from build123d import *

# Parameters (mm, degrees)
F0_R          = 19.05
F1_DEPTH      = 63.5
F3_DEPTH      = 15.875
F3_DEPTH_BACK = 4.7752
F4_R          = 6.096
F5_DEPTH      = 61.9262
F8_DEPTH      = 2.38125


with BuildPart() as f1:
    # F0 (on Front) → F1 (new body)
    with BuildSketch(Plane.XZ):
        with BuildLine():
            Line((69.85, 28.575), (0, 28.575))
            ThreePointArc((0, 28.575), (-19.345366451, -21.0306305629), (28.4756083945, 2.38125))
            ThreePointArc((28.4756083945, 2.38125), (30.9572676717, 9.6234554837), (37.9674778593, 12.7))
            Line((37.9674778593, 12.7), (69.85, 12.7))
            Line((69.85, 12.7), (69.85, 28.575))
        make_face()
        Circle(F0_R, mode=Mode.SUBTRACT)
    extrude(amount=F1_DEPTH)

    # F2 (on face) → F3 (join, two sides)
    with BuildSketch(Plane.XY.offset(28.575)) as f3_sk:
        with BuildLine():
            ThreePointArc((76.1491554441, -1.6722785358), (73.1086759125, -0.4251871176), (69.85, 0))
            ThreePointArc((69.85, 0), (60.8697438789, -3.7197438789), (57.15, -12.7))
            Line((57.15, -12.7), (57.15, -31.75))
            Line((57.15, -31.75), (57.15, -50.8))
            ThreePointArc((57.15, -50.8), (60.8697438789, -59.7802561211), (69.85, -63.5))
            ThreePointArc((69.85, -63.5), (73.1086759125, -63.0748128824), (76.1491554441, -61.8277214642))
            Line((76.1491554441, -61.8277214642), (109.4993554441, -42.7777214642))
            ThreePointArc((109.4993554441, -42.7777214642), (114.1840352623, -38.1253715915), (115.9002, -31.75))
            ThreePointArc((115.9002, -31.75), (114.1840352623, -25.3746284085), (109.4993554441, -20.7222785358))
            Line((109.4993554441, -20.7222785358), (76.1491554441, -1.6722785358))
        make_face()
    extrude(amount=-F3_DEPTH)
    extrude(f3_sk.sketch, amount=F3_DEPTH_BACK)

    # F4 (on face) → F5 (cut, through all)
    with BuildSketch(Plane.XY.offset(33.3502)):
        with Locations((69.85, -12.7)):
            Circle(F4_R)
        with Locations((69.85, -50.8)):
            Circle(F4_R)
        with Locations((103.2002, -31.75)):
            Circle(F4_R)
    extrude(amount=-F5_DEPTH, mode=Mode.SUBTRACT)

    # F7 (on offset) → F8 (join, symmetric)
    with BuildSketch(Plane.XZ.offset(31.75)):
        with BuildLine():
            ThreePointArc((28.4756083945, 2.38125), (25.7719232537, -12.3425522809), (15.9950252975, -23.6788891364))
            Line((15.9950252975, -23.6788891364), (69.85, 12.7))
            Line((69.85, 12.7), (37.9674778593, 12.7))
            ThreePointArc((37.9674778593, 12.7), (30.9572676717, 9.6234554837), (28.4756083945, 2.38125))
        make_face()
    extrude(amount=F8_DEPTH, both=True)


solid = f1.part
Input: part model. Units: mm. Frame: model coordinates. A direction names the side the tool comes from. Coordinates: 2 decimals unless noted, no trailing zeros. Loops run counter-clockwise (first coordinate to the right, second up) from the corner with the lowest first, then second, coordinate; pieces in that order, holes last.
(1) Section B-B on y = -59. Return the cut outline in (x, z) (3 decimals).
(2) Section D-D on y = -35.5. Return the cut outline in (x, z) (3 decimals), then the cut area to 3 significant figures.
(3) Pull-direction query (Y, two-part tool) for faces 1 (the face through (75.481, -53.135, 23.17)), 2 (the face through (92.591, -52.436, 22.881)), 3 (the face through (80, -31, 33.35)); classes: released by +Y, released by -Y, zero draft, split by the parting line, or undercut.
(4) Material intervals for probe 1 along Y at (x, z) = (69.85, 23.5); probe 2 along Y at (x, z) = (69, 18); probe 3 along Z at (x, y) = (21.5, -34.5) (3 decimals), sorted ascending.
(5) Section A-A on z = -2. Return the cut outline in (x, y), then the cut area to 3 significant figures.
(6) Set-up query: faces 4 (the face through (76, -31, 12.7)), 5 (the face through (42.55, -31.78, -5.74)), 6 (the face through (57.15, -31, 31)). Return all of +Z, -Z, +X, -X, +Y, -Y with unobstructed straight access to the full face (end or side cutting, diameter ignored); none if empty.
(7) First-contact query: pin 1 Ø5 at (x, y) = (20, -34) entering from +Z (3 decimals); pin 2 Ø7.5 at (x, y) = (69.85, -12.7) entering from +Z; pin 3 Ø1 at (y, z) = (-44.5, -19) entering from +X; pin 4 Ø10 at (x, y) = (17, -42) entering from -Z. Flat tips, straight axial feed; report the tip coordinate or a pass-through.
(8) Section C-C on x = 66. Return the cut outline in (y, z) (3 decimals), then the cut area to 3 significant figures.
Data:
1. outline: (0, 28.575) arc R28.575 ccw (long way) to (28.476, 2.381) arc R9.525 cw to (37.967, 12.7) - (81.1, 12.7) - (81.1, 33.35) - (60.152, 33.35) - (60.152, 28.575) - close; hole circle Ø38.1 at (0, 0)
2. outline: (0, 28.575) arc R28.575 ccw (long way) to (28.476, 2.381) arc R9.525 cw to (37.967, 12.7) - (98.394, 12.7) - (98.394, 33.35) - (57.15, 33.35) - (57.15, 28.575) - close; (108.006, 12.7) - (115.334, 12.7) - (115.334, 33.35) - (108.006, 33.35) - close; hole circle Ø38.1 at (0, 0)
2. area: 3,080 mm2
3. face 1: undercut
3. face 2: released by -Y
3. face 3: zero draft
4. probe 1: y = -63.5 to -56.9, -44.7 to -18.8, -6.6 to 0
4. probe 2: y = -63.5 to -56.84, -44.76 to -18.74, -6.66 to 0
4. probe 3: z = -18.822 to 28.575
5. outline: (-28.5, -63.5) - (-18.94, -63.5) - (-18.94, 0) - (-28.5, 0) - close; (18.94, -63.5) - (28.5, -63.5) - (28.5, -34.13) - (48.09, -34.13) - (48.09, -29.37) - (28.5, -29.37) - (28.5, 0) - (18.94, 0) - close
5. area: 1,310 mm2
6. face 4: -Z, +X
6. face 5: -Z, +X, +Y, -Y
6. face 6: +Z, -X, +Y, -Y
7. pin 1: stops at z = 28.575
7. pin 2: passes through
7. pin 3: stops at x = 21.78
7. pin 4: stops at z = -25.93
8. outline: (-63.5, 12.7) - (-55.526, 12.7) - (-55.526, 33.35) - (-62.902, 33.35) - (-62.902, 28.575) - (-63.5, 28.575) - close; (-46.074, 12.7) - (-34.131, 12.7) - (-34.131, 10.099) - (-29.369, 10.099) - (-29.369, 12.7) - (-17.426, 12.7) - (-17.426, 33.35) - (-46.074, 33.35) - close; (-7.974, 12.7) - (0, 12.7) - (0, 28.575) - (-0.598, 28.575) - (-0.598, 33.35) - (-7.974, 33.35) - close
8. area: 928 mm2
